```python
from build123d import *

# Parameters (mm, degrees)
SKETCH1_R           = 4.75
BOSS_EXTRUDE1_DEPTH = 14
CUT_EXTRUDE1_DEPTH  = 2
CUT_EXTRUDE2_DEPTH  = 2


with BuildPart() as part:
    # Sketch1 → Boss-Extrude1 (new body)
    with BuildSketch(Plane(origin=(0, 0, 0), x_dir=(1, 0, 0), z_dir=(0, 1, 0))):
        with BuildLine():
            Line((0, 9), (105, 9))
            ThreePointArc((105, 9), (107.828427125, 7.828427125), (109, 5))
            Line((109, 5), (109, -4))
            ThreePointArc((109, -4), (104.648590849, -8.957754523), (99.168268036, -5.286221686))
            ThreePointArc((99.168268036, -5.286221686), (97.78126353, -2.948377598), (95.376094526, -1.681705369))
            Line((95.376094526, -1.681705369), (72.876094526, 3.100817269))
            ThreePointArc((72.876094526, 3.100817269), (67.575536844, 0.826161371), (67.945512024, -4.929973578))
            ThreePointArc((67.945512024, -4.929973578), (68.255556035, -7.578177617), (66, -9))
            Line((66, -9), (0, -9))
            ThreePointArc((0, -9), (-9, 0), (0, 9))
        make_face()
        Circle(SKETCH1_R, mode=Mode.SUBTRACT)
    extrude(amount=BOSS_EXTRUDE1_DEPTH)

    # Sketch4 → Cut-Extrude1 (cut)
    with BuildSketch(Plane(origin=(0, 14, 0), x_dir=(1, 0, 0), z_dir=(0, 1, 0))):
        with BuildLine():
            Line((0, -8), (66, -8))
            ThreePointArc((66, -8), (67.353333621, -7.14690657), (67.167307214, -5.557984147))
            ThreePointArc((67.167307214, -5.557984147), (66.723336999, 1.349377792), (73.084006216, 4.07896487))
            Line((73.084006216, 4.07896487), (95.584006216, -0.703557768))
            ThreePointArc((95.584006216, -0.703557768), (98.470209022, -2.223564443), (100.134614429, -5.028977349))
            ThreePointArc((100.134614429, -5.028977349), (104.518872679, -7.966203618), (108, -4))
            Line((108, -4), (108, 5))
            ThreePointArc((108, 5), (107.121320344, 7.121320344), (105, 8))
            Line((105, 8), (0, 8))
            ThreePointArc((0, 8), (-8, 0), (0, -8))
        make_face()
    extrude(amount=-CUT_EXTRUDE1_DEPTH, mode=Mode.SUBTRACT)

    # Sketch5 → Cut-Extrude2 (cut)
    with BuildSketch(Plane.XZ):
        with BuildLine():
            Line((0, -8), (105, -8))
            ThreePointArc((105, -8), (107.121320344, -7.121320344), (108, -5))
            Line((108, -5), (108, 4))
            ThreePointArc((108, 4), (104.518872679, 7.966203618), (100.134614429, 5.028977349))
            ThreePointArc((100.134614429, 5.028977349), (98.470209022, 2.223564443), (95.584006216, 0.703557768))
            Line((95.584006216, 0.703557768), (73.084006216, -4.07896487))
            ThreePointArc((73.084006216, -4.07896487), (66.723336999, -1.349377792), (67.167307214, 5.557984147))
            ThreePointArc((67.167307214, 5.557984147), (67.353333621, 7.14690657), (66, 8))
            Line((66, 8), (0, 8))
            ThreePointArc((0, 8), (-8, 0), (0, -8))
        make_face()
    extrude(amount=-CUT_EXTRUDE2_DEPTH, mode=Mode.SUBTRACT)


solid = part.part
```
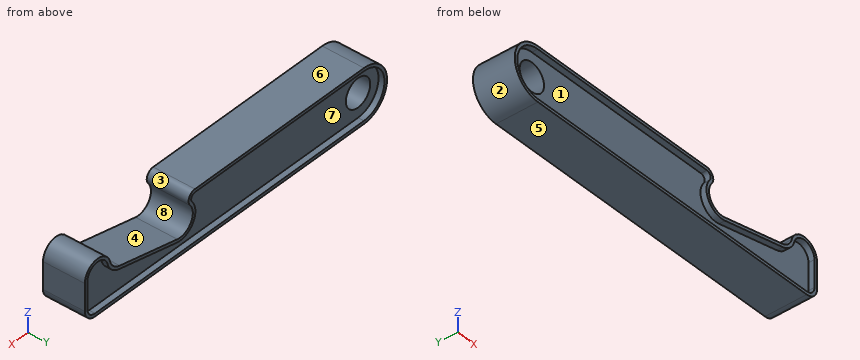
Work out the finished part from the listing and answer in its coordinate system (mm). Face numbers are marked on the shaded views. A direction names the side the tool comes from. Give positions to 0.01 mm unless a question says otherwise; leave off trailing zeros. Loops run counter-clockwise (first coordinate to the right, second up) from the corner with the lowest first, then second, coordinate; pieces in that order, holes last. Notation, with made-up numbers: (48.25, 21) -> (57.25, 21) arc R13 cw to (57.25, 41) -> close; hole circle Ø8 at (-29.75, -20.75). An arc over 180 degrees is marked (long way). One line per question, with ' | ' between items. Start each with the question number.
1) Section A-A, the plane x = 60 is taken. Determine the outline of the cut face in (y, z).
2) For the marked faces 1, 2, 3 and 4, determine the directions among +Z, -Z, +X, -X, +Y, -Y from which every point of the face is accessible in a straight line to the end or side of a thin tool.
3) Straight lines are drawn through the part: L1, parallel to Z at x = 51.5, y = 12.75; L2, parallel to X at y = 5.25, z = 3.25; L3, parallel to Y at x = 29, z = 7.75. For each, find the intervals that lie inside material, in ascending order.
4) Section C-C, the plane z = -1 is taken. Determine the outline of the cut face in (x, y).
5) Section B-B, the plane y = 7.25 is taken. Determine the outline of the cut face in (x, z).
6) Each of these flat-tipped pins is pushed along its axis until it touches: pin 1 (0.6 mm diameter, centred on y = 1.5, z = 1.5, fed in from -X); pin 2 (3 mm diameter, centred on x = 44, z = 2.5, fed in from +Y); pin 3 (4 mm diameter, centred on y = 2.5, z = 5, fed in from -X). Where does it stop, or does it pass through?
7) Determine the mould class of the marked faces 5, 6, 7 and 8 for opening direction Z: +Z half, -Z half, draft (parallel to the pull), parting line (faces both ways), or undercut.
Resolved:
1) outline: (0, -9) -> (14, -9) -> (14, -8) -> (12, -8) -> (12, 8) -> (14, 8) -> (14, 9) -> (0, 9) -> (0, 8) -> (2, 8) -> (2, -8) -> (0, -8) -> close
2) face 1: -Y | face 2: -X, +Y, -Y | face 3: +Y, -Y | face 4: +Z, +Y, -Y
3) L1: -9 to -8, 8 to 9 | L2: -8.39 to -3.46, 3.46 to 67.05, 98.07 to 109 | L3: 2 to 12
4) outline: (-8.94, 0) -> (-7.94, 0) -> (-7.94, 2) -> (-4.64, 2) -> (-4.64, 12) -> (-7.94, 12) -> (-7.94, 14) -> (-8.94, 14) -> close; (4.64, 2) -> (66.52, 2) -> (66.52, 0) -> (67.69, 0) -> (67.69, 14) -> (66.52, 14) -> (66.52, 12) -> (4.64, 12) -> close; (82.76, 0) -> (87.57, 0) -> (87.57, 2) -> (108, 2) -> (108, 0) -> (109, 0) -> (109, 14) -> (108, 14) -> (108, 12) -> (87.57, 12) -> (87.57, 14) -> (82.76, 14) -> close
5) outline: (0, -9) -> (105, -9) arc R4 ccw to (109, -5) -> (109, 4) arc R5 ccw to (99.17, 5.29) arc R5 cw to (95.38, 1.68) -> (72.88, -3.1) arc R5 cw to (67.95, 4.93) arc R2.5 ccw to (66, 9) -> (0, 9) arc R9 ccw to start; hole circle Ø9.5 at (0, 0)
6) pin 1: x = -8.92 | pin 2: y = 12 | pin 3: x = -8.49
7) face 5: -Z half | face 6: +Z half | face 7: undercut | face 8: undercut
